Design review of the part built by this model. Coordinates are the model's own, in mm. A direction names the side the tool comes from. Coordinates: 2 decimals unless noted, no trailing zeros. Loops run counter-clockwise (first coordinate to the right, second up) from the corner with the lowest first, then second, coordinate; pieces in that order, holes last. Notation, with made-up numbers: (-33, 10) - (2, 10) arc R21 ccw to (2, 15) - close; hole circle Ø7 at (0.5, 54). An arc over 180 degrees is marked (long way). One line per question, with ' | ' between items.
from build123d import *

# Parameters (mm, degrees)
SKETCH2_W           = 79.88
SKETCH2_H           = 51.8
BOSS_EXTRUDE1_DEPTH = 5.84
FILLET2_R           = 2
FILLET3_R           = 2
FILLET4_R           = 2
BOSS_EXTRUDE3_START = -3.1
BOSS_EXTRUDE3_DEPTH = 6
FILLET6_R           = 2
BOSS_EXTRUDE5_REACH = 93.015
SKETCH10_R          = 4.249482904


with BuildPart() as part:
    # Sketch2 → Boss-Extrude1 (new body)
    with BuildSketch(Plane(origin=(0, 0, 0), x_dir=(1, 0, 0), z_dir=(0, 1, 0))):
        Rectangle(SKETCH2_W, SKETCH2_H)
    extrude(amount=BOSS_EXTRUDE1_DEPTH)

    # Fillet2
    fillet2_edges = [part.edges().sort_by_distance(p)[0] for p in [
        (-39.94, 2.92, -25.9),
    ]]
    fillet(fillet2_edges, radius=FILLET2_R)

    # Fillet3
    fillet3_edges = [part.edges().sort_by_distance(p)[0] for p in [
        (-39.94, 2.92, 25.9),
    ]]
    fillet(fillet3_edges, radius=FILLET3_R)

    # Fillet4
    fillet4_edges = [part.edges().sort_by_distance(p)[0] for p in [
        (39.94, 2.92, -25.9),
    ]]
    fillet(fillet4_edges, radius=FILLET4_R)

    # Sketch3 → Boss-Extrude3 (add)
    with BuildSketch(Plane.ZY.offset(39.94).offset(BOSS_EXTRUDE3_START)):
        with BuildLine():
            Line((-22.543575681, 5.84), (22.906424319, 5.84))
            Line((22.906424319, 5.84), (22.906424319, 10.87))
            Line((22.906424319, 10.87), (18.720256409, 15.26))
            ThreePointArc((18.720256409, 15.26), (0, 51.02), (-18.720256409, 15.26))
            Line((-18.720256409, 15.26), (-22.543575681, 10.87))
            Line((-22.543575681, 10.87), (-22.543575681, 5.84))
        make_face()
    boss_extrude3 = extrude(amount=-BOSS_EXTRUDE3_DEPTH)

    # Fillet6
    fillet6_edges = [part.edges().sort_by_distance(p)[0] for p in [
        (39.94, 2.92, 25.9),
    ]]
    fillet(fillet6_edges, radius=FILLET6_R)

    # Mirror1: Boss-Extrude3 across plane
    add(boss_extrude3.mirror(Plane(origin=(0, 0, 0), x_dir=(0, 0, 1), z_dir=(1, 0, 0))))

    # Sketch10 → Boss-Extrude5 (add, up to next)
    with BuildSketch(Plane(origin=(-30.84, 0, 0), x_dir=(0, 0, -1), z_dir=(1, 0, 0)), mode=Mode.PRIVATE) as boss_extrude5_sk1:
        with Locations(Location((0, 28.24, 0), (0, 0, 180))):
            Circle(SKETCH10_R)
    boss_extrude5_tool1 = extrude(boss_extrude5_sk1.sketch, amount=BOSS_EXTRUDE5_REACH, mode=Mode.PRIVATE) - part.part
    add(boss_extrude5_tool1.solids().sort_by_distance((-30.84, 28.24, 0))[0])


solid = part.part
Q1. Draft analysis for pull direction X (two halves, no side actions). For faces 6 (the flat face through (-30.84, 23.7, -0.3)), 7 (the flat face through (33.9, 13.1, -20.6)), 8 (the flat face through (30.84, 23.7, -0.3)), 9 (the flat face through (-39.94, 3, 0)), state which applies: +X half, -X half, draft (parallel to the pull), parting line (faces both ways), or undercut.
Returned:
face 6: undercut | face 7: draft | face 8: undercut | face 9: -X half
Q2. Take a section at D-D (y = 28.24). Give the boundary of the cut face in (x, z), plus the area to 3 significant figures.
Returned:
outline: (-36.84, -22.78) - (-30.84, -22.78) - (-30.84, -4.25) - (30.84, -4.25) - (30.84, -22.78) - (36.84, -22.78) - (36.84, 22.78) - (30.84, 22.78) - (30.84, 4.25) - (-30.84, 4.25) - (-30.84, 22.78) - (-36.84, 22.78) - close | area: 1,070 mm²
Q3. Take a section at B-B (x = -17). Give the boundary of the cut face in (y, z), plus the area to 3 significant figures.
Returned:
outline: (0, -25.9) - (5.84, -25.9) - (5.84, 25.9) - (0, 25.9) - close; circle Ø8.5 at (28.24, 0) | area: 359 mm²
Q4. For pin 1 (1.5 mm diameter, centred on x = -32.5, y = 7.5, fed in from +Z); pin 2 (1.5 mm diameter, centred on x = 25, z = 11.5, fed in from +Y); pin 3 (2.5 mm diameter, centred on x = 34.5, y = 8.5, fed in from -Z), all flat-tipped, find the tip position at first contact; note any pin that passes through.
Returned:
pin 1: stops at z = 22.91 | pin 2: stops at y = 5.84 | pin 3: stops at z = -22.54
Q5. Tool access review of faces 1 (the flat face through (34, 8, -22.544)), 2 (the flat face through (36.84, 29, 0)), 3 (the flat face through (34, 8, 22.906)), 4 (the cylindrical face through (34, 51, 1)), 5 (the flat face through (33.882, 13.034, 20.843)): name each direction out of +Z, -Z, +X, -X, +Y, -Y from which nothing blocks a thin tool from reaching the whole face with its end or side.
Returned:
face 1: -Z, +X, -X | face 2: +Z, -Z, +X, +Y | face 3: +Z, +X, -X, +Y | face 4: +X, -X | face 5: +Z, +X, -X
Q6. To check wall thickness, follow line 1 along X through (y, z) = (31.5, -7); line 2 along Y through (x, z) = (-16.5, -10); line 3 along Z through (x, y) = (2.5, 28). State the ranges of each line that lie inside material, in increasing order.
Returned:
line 1: x = -36.84 to -30.84, 30.84 to 36.84 | line 2: y = 0 to 5.84 | line 3: z = -4.24 to 4.24
Q7. Take a section at C-C (z = 20). Give the boundary of the cut face in (x, y).
Returned:
outline: (-39.94, 0) - (39.94, 0) - (39.94, 5.84) - (36.84, 5.84) - (36.84, 13.92) - (30.84, 13.92) - (30.84, 5.84) - (-30.84, 5.84) - (-30.84, 13.92) - (-36.84, 13.92) - (-36.84, 5.84) - (-39.94, 5.84) - close; (-36.84, 17.33) - (-30.84, 17.33) - (-30.84, 39.15) - (-36.84, 39.15) - close; (30.84, 17.33) - (36.84, 17.33) - (36.84, 39.15) - (30.84, 39.15) - close
Q8. Take a section at A-A (z = 0). Give the boundary of the cut face in (x, y).
Returned:
outline: (-39.94, 0) - (39.94, 0) - (39.94, 5.84) - (36.84, 5.84) - (36.84, 51.02) - (30.84, 51.02) - (30.84, 32.49) - (-30.84, 32.49) - (-30.84, 51.02) - (-36.84, 51.02) - (-36.84, 5.84) - (-39.94, 5.84) - close; hole (-30.84, 5.84) - (30.84, 5.84) - (30.84, 23.99) - (-30.84, 23.99) - close
